Check sheet for the drawn part. Datum: minimum x, y, z corner. Units: mm. A direction names the side the tool comes from. Give positions to 0.01 mm unless a question says otherwise; leave off trailing zeros. Write each loop counter-clockwise with the first axis right and the second up, starting at its lowest first coordinate (ties: lowest second). Pieces come first, ordered by that corner, then holes. Notation, with made-up numbers: (-16, 71.5) - (-4, 71.5) arc R16 cw to (-4, 78.5) - close; hole circle Ø9 at (79.5, -23). An arc over 180 degrees is marked (long way). Return JSON: item names as keys, results as strings. Group by question number.
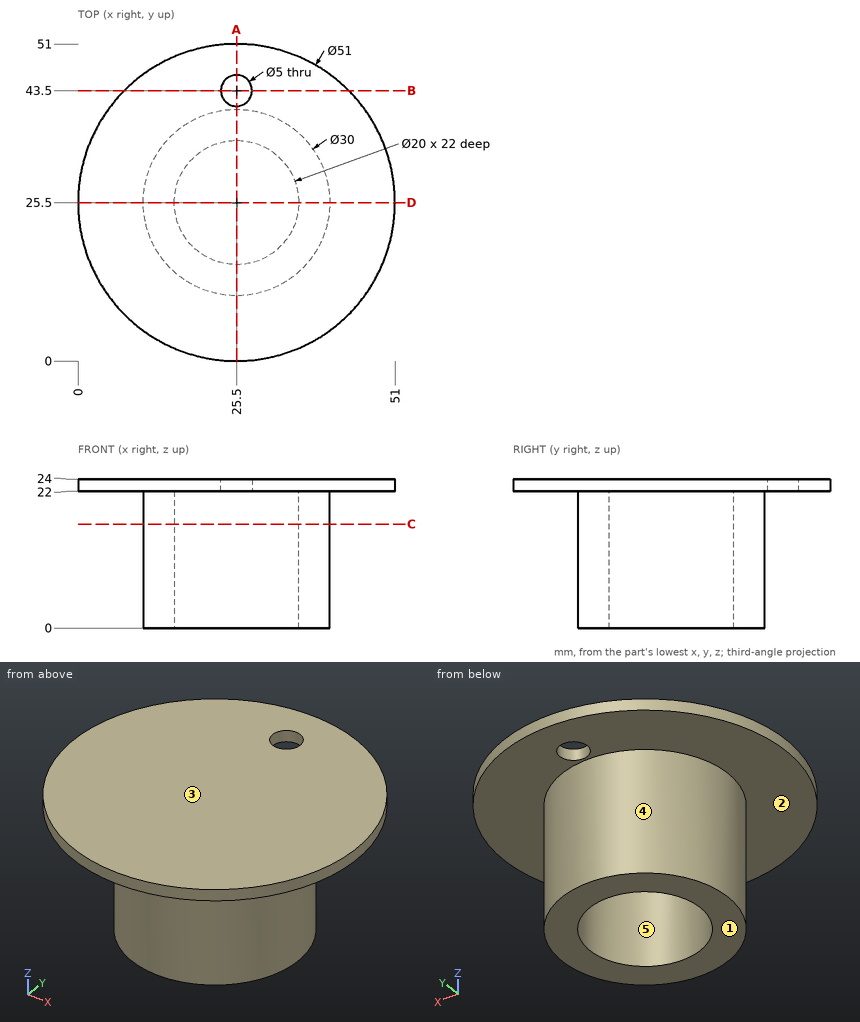
Item 1: Section check C-C on z = 16.75. Record the cut outline in (x, y), plus the area to 3 significant figures.
Item 2: Section check A-A on x = 25.5. Record the cut outline in (y, z), plus the area to 3 significant figures.
Item 3: Section check D-D on y = 25.5. Record the cut outline in (x, z).
Item 4: Access from +Z, -Z, +X, -X, +Y, -Y to the whole of each face (thin tool, end or side, straight path). Record for the marked faces 1 and 2.
Item 5: Mould release check, pull along X, two halves, no side actions. Record for the marked faces 3, 4 and 5: +X half, -X half, draft (parallel to the pull), parting line (faces both ways), or undercut.
Item 6: Section check B-B on y = 43.5. Record the cut outline in (x, z).
Item 7: Depth check by flat-ended pin: pin 1 (1 mm diameter, centred on x = 15, y = 43.5, fed in from -Z); pin 2 (3 mm diameter, centred on y = 35.5, z = 13.5, fed in from -X); pin 3 (8 mm diameter, centred on x = 42.5, z = 18.5, fed in from +Y). Enter the tip coordinate at first touch or a pass-through.
Item 8: Material ranges on line 1 along Y through (x, z) = (25.5, 8.5); line 2 along Y through (x, z) = (25.5, 22.8); line 3 along Z through (x, y) = (5, 22.5), recorded low to high. Write a range as from..to.
Reply:
{
 "1": {"outline": "circle Ø30 at (25.5, 25.5); hole circle Ø20 at (25.5, 25.5)", "area": "393 mm²"},
 "2": {"outline": "(0, 22) - (10.5, 22) - (10.5, 0) - (15.5, 0) - (15.5, 22) - (35.5, 22) - (35.5, 0) - (40.5, 0) - (40.5, 22) - (41, 22) - (41, 24) - (0, 24) - close; (46, 22) - (51, 22) - (51, 24) - (46, 24) - close", "area": "312 mm²"},
 "3": {"outline": "(0, 22) - (10.5, 22) - (10.5, 0) - (15.5, 0) - (15.5, 22) - (35.5, 22) - (35.5, 0) - (40.5, 0) - (40.5, 22) - (51, 22) - (51, 24) - (0, 24) - close"},
 "4": {"face 1": "-Z, +X, -X, +Y, -Y", "face 2": "-Z"},
 "5": {"face 3": "draft", "face 4": "parting line", "face 5": "undercut"},
 "6": {"outline": "(7.44, 22) - (23, 22) - (23, 24) - (7.44, 24) - close; (28, 22) - (43.56, 22) - (43.56, 24) - (28, 24) - close"},
 "7": {"pin 1": "z = 22", "pin 2": "x = 13.14", "pin 3": "y = 46.08"},
 "8": {"line 1": "10.5..15.5, 35.5..40.5", "line 2": "0..41, 46..51", "line 3": "22..24"}
}
